Part model, mm, in its own coordinate system. Round coordinates to 2 decimals unless told otherwise and drop trailing zeros. Use a Markdown table: item, result. Add a question column.
1) Wall check: probe 1 along Y at (x, z) = (-174, 2.3); probe 2 along Y at (x, z) = (-22.5, 1.5); probe 3 along Z at (x, y) = (-166, 0.25) (3 decimals). Give the ranges that are in metal, low to high.
2) Two-plate mould, pull along X, no slides. Class faces 1 (the face through (-200, -0.3, -0.2)), 2 (the face through (0, -0.3, -0.2)), 3 (the face through (-99, 0, -0.405)): released by +X, released by -X, zero draft, split by the parting line, or undercut.
3) Drop flat-ended pins along their axis: P1, Ø1, axis at x = -76.5, z = 2, coming from the +Y side; P2, Ø0.8, axis at x = -135.5, z = 1, coming from the +Y side; P3, Ø1.5, axis at y = 1.5, z = 0.5, coming from the +X side; P4, Ø0.5, axis at x = -85, z = 2.5, coming from the -Y side. Give the stop position or say it passes through.
Autodesk Fusion 360 part; units mm, degrees
sketch "Sketch1" plane through (0, 0, 0) normal (1, 0, 0) x (0, 1, 0) in component "Cover"
sketch "Sketch2" plane through (0, 0, 0) normal (1, 0, 0) x (0, 1, 0) in component "Cover"
  line L0 (-3.5, -0.405) -> (3.5, -0.405)
  line L1 (-3.5, -0.405) -> (-3.5, -0.005)
  line L2 (3.5, -0.405) -> (3.5, -0.005)
  line L3 (-3, -0.005) -> (-3, 1.895)
  line L4 (3, -0.005) -> (3, 1.895)
  line L5 (-1.8, -0.005) -> (-1.8, 1.895)
  line L6 (1.8, -0.005) -> (1.8, 1.895)
  line L7 (-1.8, 1.895) -> (-1.8, 2.795)
  line L8 (1.8, 1.895) -> (1.8, 2.795)
  line L9 (-1.8, 2.795) -> (-3.2, 2.795)
  line L10 (1.8, 2.795) -> (3.2, 2.795)
  line L11 (-3, 1.895) -> (-3.2, 1.895)
  line L12 (3, 1.895) -> (3.2, 1.895)
  line L13 (-3.2, 2.795) -> (-3.2, 1.895)
  line L14 (3.2, 2.795) -> (3.2, 1.895)
  line L15 (-3.5, -0.005) -> (-3, -0.005)
  line L16 (-1.8, -0.005) -> (1.8, -0.005)
  line L17 (3, -0.005) -> (3.5, -0.005)
  dimension "d6" = 7
  dimension "d10" = 0.4
  dimension "d12" = 0.4
  dimension "d13" = 3
  dimension "d14" = 3
  dimension "d17" = 1.9
  dimension "d18" = 1.9
  dimension "d20" = 1.2
  dimension "d21" = 1.2
  dimension "d25" = 1.4
  dimension "d26" = 0.2
  dimension "d39" = 2.8
  dimension "d40" = 0.005
  dimension "d41" = 3.5
extrude "Extrude1" add sketch "Sketch2" against normal blind 200 in component "Cover"
fillet "Fillet1" radius 1 1 edges at (-100, 1.8, -0.005) in component "Cover"
fillet "Fillet2" radius 1 1 edges at (-100, -1.8, -0.005) in component "Cover"
chamfer "Chamfer1" distance 0.2 angle 45 1 edges at (-100, 3.2, 1.895) in component "Cover"
chamfer "Chamfer2" distance 0.2 angle 45 1 edges at (-100, -3.2, 1.895) in component "Cover"
fillet "Fillet3" radius 0.2 1 edges at (-100, -3, -0.005) in component "Cover"
fillet "Fillet4" radius 0.2 1 edges at (-100, 3, -0.005) in component "Cover"
chamfer "Chamfer3" distance 0.3 angle 45 2 edges at (-100, -3.2, 2.795) (-100, 3.2, 2.795) in component "Cover"
component "Cover" placed x (1, 0, 0) y (0, 1, 0) z (0, 0, 1) at (0, 0, 0)
equation "width_bottom = 7 mm"
equation "Bottom_radius = 0.2 mm"
equation "radius_inside = 1 mm"
equation "chamfer_inside = 0.2 mm"
equation "length = 200 mm"
equation "d6 = width_bottom"
equation "layer_height = 0.2 mm"
equation "d10 = num_layer_bottom * layer_height"
equation "d12 = num_layer_bottom * layer_height"
equation "height_below_chamfer = 1.9 mm"
equation "chamfe_angle = 60 deg"
equation "d17 = height_below_chamfer"
equation "d18 = height_below_chamfer"
equation "wall_width = 1.2 mm"
equation "d20 = wall_width"
equation "d21 = wall_width"
equation "overhang = 0.2 mm"
equation "height_overall = 2.8 mm"
equation "d25 = wall_width + overhang"
equation "d26 = overhang"
equation "d30 = radius_inside"
equation "d32 = radius_inside"
equation "d33 = chamfer_inside"
equation "d34 = chamfer_inside"
equation "d36 = Bottom_radius"
equation "d38 = Bottom_radius"
equation "d39 = height_overall"
equation "d41 = width_bottom / 2"
Entries:
| question | item | result |
|---|---|---|
| 1 | probe 1 | y = -3.2 to -1.8, 1.8 to 3.2 |
| 1 | probe 2 | y = -3 to -1.8, 1.8 to 3 |
| 1 | probe 3 | z = -0.405 to -0.005 |
| 2 | face 1 | released by -X |
| 2 | face 2 | released by +X |
| 2 | face 3 | zero draft |
| 3 | P1 | stops at y = 3.2 |
| 3 | P2 | stops at y = 3 |
| 3 | P3 | stops at x = 0 |
| 3 | P4 | stops at y = -3.2 |
